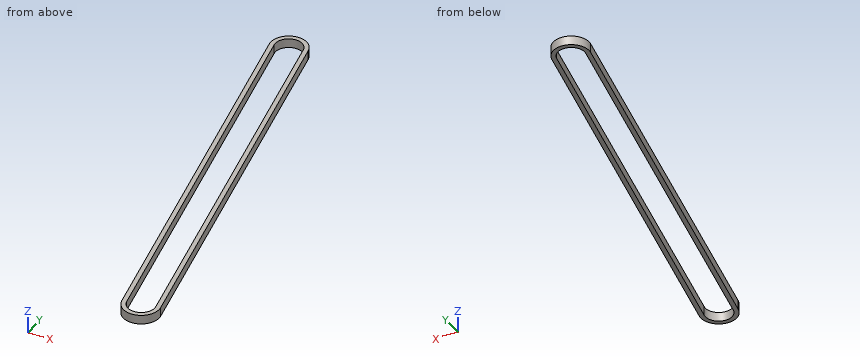
from build123d import *

# Parameters (mm, degrees)
BOSS_EXTRUDE1_DEPTH = 4
CUT_EXTRUDE1_DEPTH  = 4


with BuildPart() as part:
    # Sketch3 → Boss-Extrude1 (new body)
    with BuildSketch(Plane.XY):
        with BuildLine():
            Line((44.988998007, -182.443553074), (7.742974777, 1.567272025))
            ThreePointArc((7.742974777, 1.567272025), (-1.567272025, 7.742974777), (-7.742974777, -1.567272025))
            Line((-7.742974777, -1.567272025), (29.503048453, -185.578097123))
            ThreePointArc((29.503048453, -185.578097123), (38.813295255, -191.753799876), (44.988998007, -182.443553074))
        make_face()
    extrude(amount=BOSS_EXTRUDE1_DEPTH)

    # Sketch4 → Cut-Extrude1 (cut)
    with BuildSketch(Plane.XY.offset(4)):
        with BuildLine():
            Line((43.028751228, -182.840330802), (5.782727998, 1.170494297))
            ThreePointArc((5.782727998, 1.170494297), (-1.170494297, 5.782727998), (-5.782727998, -1.170494297))
            Line((-5.782727998, -1.170494297), (31.463295232, -185.181319396))
            ThreePointArc((31.463295232, -185.181319396), (38.416517527, -189.793553097), (43.028751228, -182.840330802))
        make_face()
    extrude(amount=-CUT_EXTRUDE1_DEPTH, mode=Mode.SUBTRACT)


solid = part.part
Design review of the part built by this model. Coordinates are the model's own, in mm. Give positions to 0.01 mm unless a question says otherwise; leave off trailing zeros. Loops run counter-clockwise (first coordinate to the right, second up) from the corner with the lowest first, then second, coordinate; pieces in that order, holes last. Notation, with made-up numbers: (-39.5, 18.25) -> (-5.5, 18.25) arc R4 ccw to (-5.5, 24.25) -> close; hole circle Ø4 at (-28.75, 38.5). An arc over 180 degrees is marked (long way). One line per question, with ' | ' between items. Start each with the question number.
(1) We need section B-B (y = -95.5). State the section outline as (x, z) points.
(2) For line 1 (X direction, y = -20, z = 1.4); line 2 (X direction, y = -146, z = 1.05), list the stretches that pass through material, from the lowest coordinate up.
(3) We need section A-A (z = 0.75). State the section outline as (x, y) points.
(4) We need section C-C (x = 0). State the section outline as (y, z) points.
(5) Insertion check: P1, Ø1, axis at y = -125.5, z = 1.5, coming from the -X side; P2, Ø1.5, axis at x = -1.5, z = 3.5, coming from the +Y side. Each pin has a flat end and moves straight along its axis. Give the tip position at first contact, or say it passes through.
The answers:
1) outline: (11.27, 0) -> (13.31, 0) -> (13.31, 4) -> (11.27, 4) -> close; (25.35, 0) -> (27.39, 0) -> (27.39, 4) -> (25.35, 4) -> close
2) line 1: x = -4.01 to -1.97, 10.07 to 12.11 | line 2: x = 21.49 to 23.53, 35.57 to 37.61
3) outline: (-7.74, -1.57) -> (29.5, -185.58) arc R7.9 ccw to (44.99, -182.44) -> (7.74, 1.57) arc R7.9 ccw to start; hole (-5.78, -1.17) -> (31.46, -185.18) arc R5.9 ccw to (43.03, -182.84) -> (5.78, 1.17) arc R5.9 ccw to start
4) outline: (-39.82, 0) -> (-29.74, 0) -> (-29.74, 4) -> (-39.82, 4) -> close; (5.9, 0) -> (7.9, 0) -> (7.9, 4) -> (5.9, 4) -> close
5) P1: stops at x = 17.24 | P2: stops at y = 7.86
